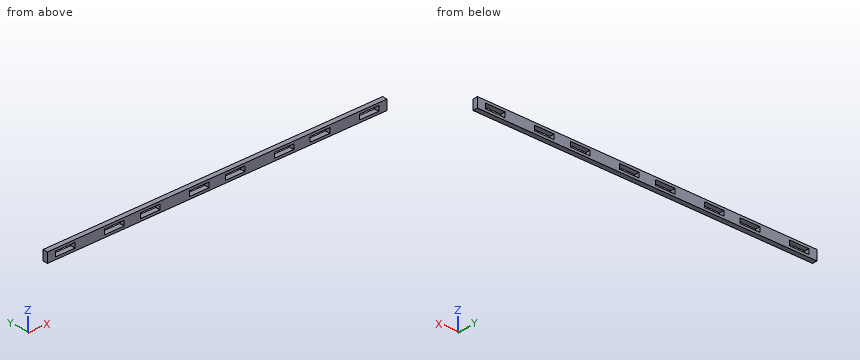
from build123d import *

# Parameters (mm, degrees)
SKETCH1_W           = 439.940905232
SKETCH1_H           = 12.7
BOSS_EXTRUDE1_DEPTH = 6.35
SKETCH2_W           = 25.4
SKETCH2_H           = 6.35
CUT_EXTRUDE1_DEPTH  = 7.35
LPATTERN1_COUNT     = 2
LPATTERN1_PITCH     = 219.970452616
LPATTERN1_COL_COUNT = 2
LPATTERN1_COL_PITCH = 219.970452616


with BuildPart() as part:
    # Sketch1 → Boss-Extrude1 (new body)
    with BuildSketch(Plane(origin=(0, 0, 0), x_dir=(1, 0, 0), z_dir=(0, 1, 0))):
        Rectangle(SKETCH1_W, SKETCH1_H)
    extrude(amount=BOSS_EXTRUDE1_DEPTH)

    # Sketch2 → Cut-Extrude1 (cut, through all)
    with BuildSketch(Plane(origin=(0, 6.35, 0), x_dir=(1, 0, 0), z_dir=(0, 1, 0))):
        with Locations((-23.242613154, 0)):
            Rectangle(SKETCH2_W, SKETCH2_H)
        with Locations((23.242613154, 0)):
            Rectangle(SKETCH2_W, SKETCH2_H)
        with Locations((-86.742613154, 0)):
            Rectangle(SKETCH2_W, SKETCH2_H)
        with Locations((86.742613154, 0)):
            Rectangle(SKETCH2_W, SKETCH2_H)
    cut_extrude1 = extrude(amount=-CUT_EXTRUDE1_DEPTH, mode=Mode.SUBTRACT)

    # LPattern1: Cut-Extrude1 ×2
    with Locations(*[(i * LPATTERN1_PITCH, 0, 0) for i in range(1, LPATTERN1_COUNT)]):
        add(cut_extrude1, mode=Mode.SUBTRACT)

    # LPattern1 col: Cut-Extrude1 ×2
    with Locations(*[(-i * LPATTERN1_COL_PITCH, 0, 0) for i in range(1, LPATTERN1_COL_COUNT)]):
        add(cut_extrude1, mode=Mode.SUBTRACT)


solid = part.part
Input: part model. Units: mm. Frame: model coordinates. Give positions to 0.01 mm unless a question says otherwise; leave off trailing zeros. Write each loop counter-clockwise with the first axis right and the second up, starting at its lowest first coordinate (ties: lowest second). Pieces come first, ordered by that corner, then holes.
Q1. Section B-B, the plane y = 1.75. State how many separate pieces and enclosed holes the cut face has, plus the area to 3 significant figures.
Q2. Material intervals for probe 1 along Z at (x, y) = (23, 3) (3 decimals), sorted ascending.
Q3. Section A-A, the plane x = -26.5. Output: boundary loops of the cut face in (y, z) (3 decimals), plus the area to 3 significant figures.
Filled in:
1. separate pieces: 1
1. enclosed holes: 8
1. area: 4,300 mm2
2. probe 1: z = -6.35 to -3.175, 3.175 to 6.35
3. outline: (0, -6.35) - (6.35, -6.35) - (6.35, -3.175) - (0, -3.175) - close; (0, 3.175) - (6.35, 3.175) - (6.35, 6.35) - (0, 6.35) - close
3. area: 40.3 mm2
